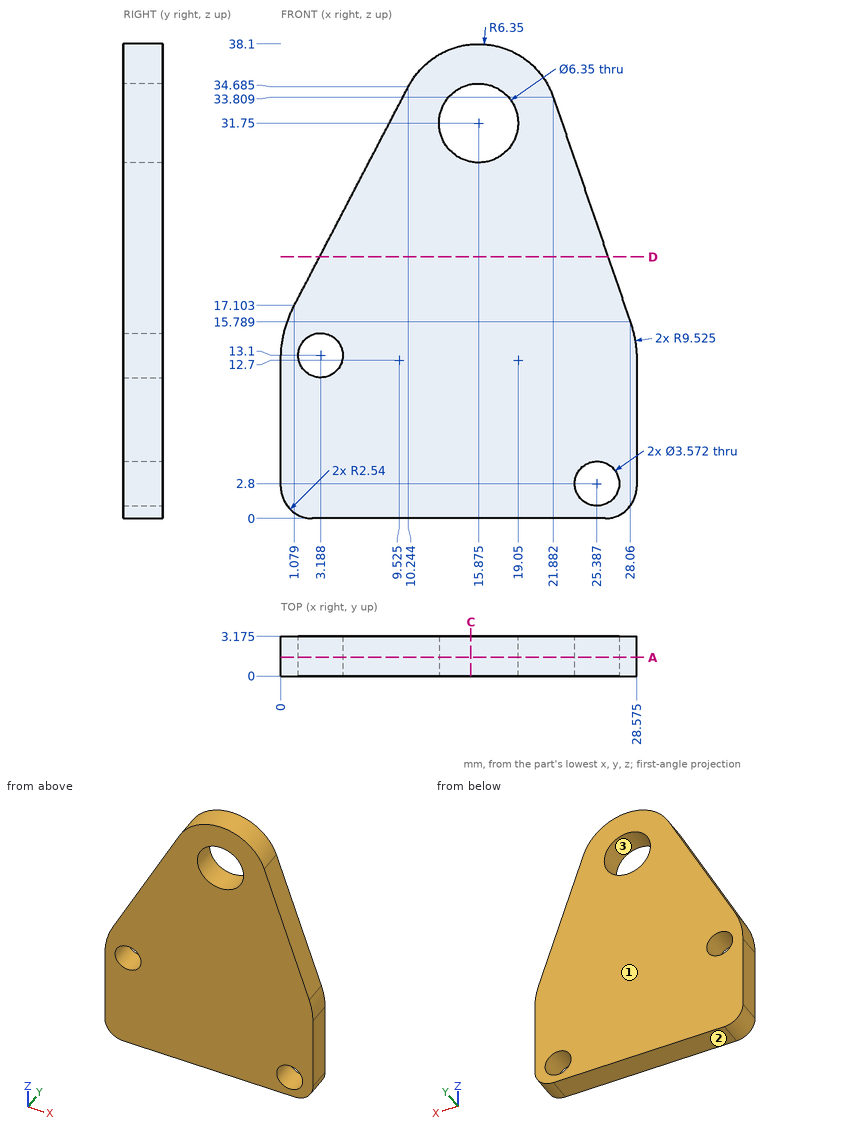
Check sheet for the drawn part. Datum: minimum x, y, z corner. Units: mm. Give positions to 0.01 mm unless a question says otherwise; leave off trailing zeros. Order: outer loops, then holes, each group sorted by start corner. A loop starts at its lowest first (then second) coordinate and runs counter-clockwise, first axis right, second up. Notation, with made-up numbers: (27, 27.5) - (48, 27.5) arc R20 ccw to (48, 36.5) - close; hole circle Ø3 at (63, 81). An arc over 180 degrees is marked (long way). Answer in a Markdown table with one row per item. Add a question column.
Q1. Cross-section at C-C, the plane x = 15.25. Enter the section's corners in (y, z) (1 decimal), then the cut area to 3 significant figures.
Q2. Mould release check, pull along Z, two halves, no side actions. Record for the marked faces 1, 2 and 3: pulls with the +Z half, pulls with the -Z half, needs draft (parallel to the pull), parting line crosses it, or undercut.
Q3. Material ranges on probe 1 along Z at (x, y) = (15, 2.15); probe 2 along Z at (x, y) = (15.5, 1.8); probe 3 along X at (y, z) = (0.45, 30.5) (1 decimal), recorded low to high. Write a range as from..to.
Q4. Cross-section at D-D, the plane z = 21. Enter the section's corners in (x, y) (1 decimal).
Q5. Gauge pin test, flat ends, axial feed: pin 1 (3 mm diameter, centred on x = 25.39, z = 2.8, fed in from +Y); pin 2 (1.5 mm diameter, centred on y = 1, z = 23, fed in from -X); pin 3 (1 mm diameter, centred on x = 3.5, y = 0.5, fed in from +Z) (1 decimal). Record the tip position at first contact, or that the pin passes through.
Q6. Cross-section at A-A, the plane y = 1.5. Count the separate pieces of the cut face and the enclosed holes in it.
Check values:
| question | item | result |
|---|---|---|
| 1 | outline | (0, 0) - (3.2, 0) - (3.2, 28.6) - (0, 28.6) - close; (0, 34.9) - (3.2, 34.9) - (3.2, 38.1) - (0, 38.1) - close |
| 1 | area | 101 mm^2 |
| 2 | face 1 | needs draft |
| 2 | face 2 | pulls with the -Z half |
| 2 | face 3 | undercut |
| 3 | probe 1 | z = 0..28.7, 34.8..38.04 |
| 3 | probe 2 | z = 0..28.6, 34.9..38.09 |
| 3 | probe 3 | x = 8.1..13, 18.8..23 |
| 4 | outline | (3.1, 0) - (26.3, 0) - (26.3, 3.2) - (3.1, 3.2) - close |
| 5 | pin 1 | passes through |
| 5 | pin 2 | stops at x = 3.76 |
| 5 | pin 3 | stops at z = 22.7 |
| 6 | separate pieces | 1 |
| 6 | enclosed holes | 3 |
